For this review, take the finished solid that the model builds, in its own axes (mm). Face numbers are marked on the shaded views. A direction names the side the tool comes from. Round coordinates to 2 decimals unless told otherwise and drop trailing zeros. Write each loop counter-clockwise with the first axis right and the second up, starting at its lowest first coordinate (ties: lowest second). Pieces come first, ordered by that corner, then holes. Notation, with made-up numbers: M 76,85.5 L 89,85.5 A24 cw 89,110.5 Z; hole C -35.5,-0.5 d5. An arc over 180 degrees is marked long. Use one line per item in the form item = value. Start each with the question number.
Item 1: For P1, Ø2.5, axis at x = 18, y = 17, coming from the +Z side; P2, Ø6, axis at y = 10, z = 50.5, coming from the -X side; P3, Ø2.5, axis at x = 15.5, y = -15.5, coming from the +Z side; P4, Ø10, axis at y = 8.5, z = 47, coming from the -X side, all flat-tipped, find the tip position at first contact; note any pin that passes through.
Item 2: For line 1 (X direction, y = -17, z = 7); line 2 (Y direction, x = 19, z = 39.5); line 3 (X direction, y = -17.5, z = 49.5), list the stretches that pass through material, from the lowest coordinate up. Write a range as [from, to].
Item 3: Add section B-B (y = 9). State the section outline as (x, z) points, and give its area (3 significant figures).
Item 4: Draft analysis for pull direction Z (two halves, no side actions). For the marked faces 1, 2 and 3, state which applies: released by +Z, released by -Z, zero draft, split by the parting line, or undercut.
Item 5: Add section D-D (y = -15.5). State the section outline as (x, z) points, and give its area (3 significant figures).
Item 6: Add section A-A (z = 27). State the section outline as (x, y) points.
Item 7: For the marked faces 4, 5 and 6, list the 3-axis set-ups (+Z, -Z, +X, -X, +Y, -Y) from which the entire face can be reached by the end or side of a thin tool; tool diameter is ignored.
Item 8: Add section C-C (z = 10.5). State the section outline as (x, y) points, and give its area (3 significant figures).
from build123d import *

# Parameters (mm, degrees)
SKETCH1_W           = 42
SKETCH1_H           = 42
BOSS_EXTRUDE1_DEPTH = 9.5
CHAMFER1_SIZE       = 4.5
BOSS_EXTRUDE2_DEPTH = 22.2
FILLET1_R           = 1
BOSS_EXTRUDE3_DEPTH = 11
SKETCH5_R           = 21
BOSS_EXTRUDE4_DEPTH = 28


with BuildPart() as part:
    # Sketch1 → Boss-Extrude1 (new body)
    with BuildSketch(Plane.XY):
        Rectangle(SKETCH1_W, SKETCH1_H)
    extrude(amount=-BOSS_EXTRUDE1_DEPTH)

    # Chamfer1
    chamfer1_edges = [part.edges().sort_by_distance(p)[0] for p in [
        (21, -21, -4.75),
        (-21, -21, -4.75),
        (-21, 21, -4.75),
        (21, 21, -4.75),
    ]]
    chamfer(chamfer1_edges, length=CHAMFER1_SIZE)

    # Sketch3 → Boss-Extrude2 (add)
    with BuildSketch(Plane.XY):
        Polygon((13.5, 21), (-13.5, 21), (-21, 13.5), (-21, -13.5), (-13.5, -21), (13.5, -21), (21, -13.5), (21, 13.5), align=None)
    extrude(amount=BOSS_EXTRUDE2_DEPTH)

    # Fillet1
    fillet1_edges = [part.edges().sort_by_distance(p)[0] for p in [
        (-13.5, 21, 11.1),
        (-21, 13.5, 11.1),
        (-21, -13.5, 11.1),
        (-13.5, -21, 11.1),
        (13.5, -21, 11.1),
        (21, -13.5, 11.1),
        (21, 13.5, 11.1),
        (13.5, 21, 11.1),
    ]]
    fillet(fillet1_edges, radius=FILLET1_R)

    # Sketch4 → Boss-Extrude3 (add)
    with BuildSketch(Plane.XY.offset(22.2)):
        Polygon((-21, 16.5), (-16.5, 21), (16.5, 21), (21, 16.5), (21, -16.5), (16.5, -21), (-16.5, -21), (-21, -16.5), align=None)
    extrude(amount=BOSS_EXTRUDE3_DEPTH)

    # Sketch5 → Boss-Extrude4 (add)
    with BuildSketch(Plane.XY.offset(33.2)):
        Circle(SKETCH5_R)
    extrude(amount=BOSS_EXTRUDE4_DEPTH)


solid = part.part
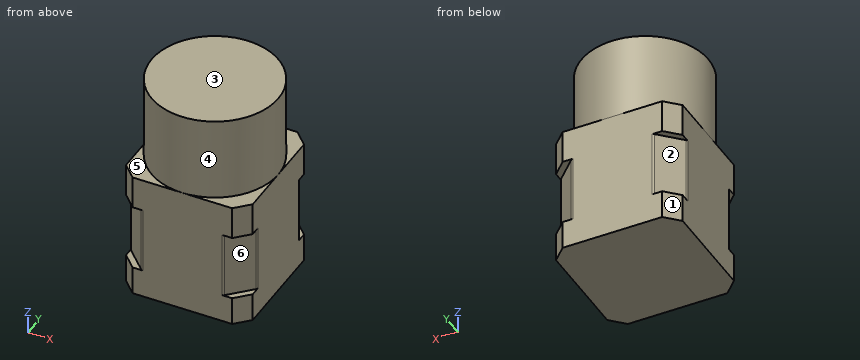
Calculated:
q1.P1 = 33.2
q1.P2 = -19.8
q1.P3 = 61.2
q1.P4 = -20.71
q2.line_1 = [-17.5, 17.5]
q2.line_2 = [-8.94, 8.94]
q2.line_3 = [-11.61, 11.61]
q3.outline = M -21,-9.5 L 21,-9.5 L 21,33.2 L 18.97,33.2 L 18.97,61.2 L -18.97,61.2 L -18.97,33.2 L -21,33.2 Z
q3.area = 2,860 mm^2
q4.face_1 = zero draft
q4.face_2 = undercut
q4.face_3 = released by +Z
q5.outline = M -21,-9.5 L 21,-9.5 L 21,0 L 19,0 L 19,22.2 L 21,22.2 L 21,33.2 L 14.17,33.2 L 14.17,61.2 L -14.17,61.2 L -14.17,33.2 L -21,33.2 L -21,22.2 L -19,22.2 L -19,0 L -21,0 Z
q5.area = 2,500 mm^2
q6.outline = M -21,-16.5 L -16.5,-21 L 16.5,-21 L 21,-16.5 L 21,16.5 L 16.5,21 L -16.5,21 L -21,16.5 Z
q7.face_4 = +Z
q7.face_5 = +Z, -X, -Y
q7.face_6 = +X, -Y
q8.outline = M -21,-13.09 A1 ccw -20.71,-13.79 L -13.79,-20.71 A1 ccw -13.09,-21 L 13.09,-21 A1 ccw 13.79,-20.71 L 20.71,-13.79 A1 ccw 21,-13.09 L 21,13.09 A1 ccw 20.71,13.79 L 13.79,20.71 A1 ccw 13.09,21 L -13.09,21 A1 ccw -13.79,20.71 L -20.71,13.79 A1 ccw -21,13.09 Z
q8.area = 1,650 mm^2
